from build123d import *

# Parameters (mm, degrees)
SKETCH1_R           = 21.5
SKETCH1_R_2         = 5
BOSS_EXTRUDE1_DEPTH = 5
EXTRUDE_THIN1_START = -100
SKETCH2_R           = 26.5
SKETCH2_R_2         = 21.5
EXTRUDE_THIN1_DEPTH = 100
CUT_EXTRUDE1_DEPTH  = 50
BOSS_EXTRUDE2_DEPTH = 5
SKETCH5_R           = 6
CUT_EXTRUDE2_DEPTH  = 5


with BuildPart() as part:
    # Sketch1 → Boss-Extrude1 (new body)
    with BuildSketch(Plane.XY):
        Circle(SKETCH1_R)
        Circle(SKETCH1_R_2, mode=Mode.SUBTRACT)
    extrude(amount=BOSS_EXTRUDE1_DEPTH)

    # Sketch2 → Extrude-Thin1 (add)
    with BuildSketch(Plane.XY.offset(5).offset(EXTRUDE_THIN1_START)):
        Circle(SKETCH2_R)
        Circle(SKETCH2_R_2, mode=Mode.SUBTRACT)
    extrude(amount=EXTRUDE_THIN1_DEPTH)

    # Sketch3 → Cut-Extrude1 (cut)
    with BuildSketch(Plane(origin=(0, 0, -95), x_dir=(-1, 0, 0), z_dir=(0, 0, -1))):
        with BuildLine():
            Line((11.936744149, -23.659335137), (11.494827009, -18.169175876))
            ThreePointArc((11.494827009, -18.169175876), (21.430686769, 1.725011487), (8.440695566, 19.773837725))
            Line((8.440695566, 19.773837725), (7.998778427, 25.263996985))
            ThreePointArc((7.998778427, 25.263996985), (26.414567412, 2.126176949), (11.936744149, -23.659335137))
        make_face()
        with BuildLine():
            Line((-11.494827009, 18.169175876), (-11.936744149, 23.659335137))
            ThreePointArc((-11.936744149, 23.659335137), (-26.414567412, -2.126176949), (-7.998778427, -25.263996985))
            Line((-7.998778427, -25.263996985), (-8.440695566, -19.773837725))
            ThreePointArc((-8.440695566, -19.773837725), (-21.430686769, -1.725011487), (-11.494827009, 18.169175876))
        make_face()
    extrude(amount=-CUT_EXTRUDE1_DEPTH, mode=Mode.SUBTRACT)

    # Sketch4 → Boss-Extrude2 (add)
    with BuildSketch(Plane(origin=(0, 0, -95), x_dir=(-1, 0, 0), z_dir=(0, 0, -1))):
        with BuildLine():
            Line((-11.494827009, 18.169175876), (-8.440695566, -19.773837725))
            ThreePointArc((-8.440695566, -19.773837725), (1.725011487, -21.430686769), (11.494827009, -18.169175876))
            Line((11.494827009, -18.169175876), (8.440695566, 19.773837725))
            ThreePointArc((8.440695566, 19.773837725), (-1.725011487, 21.430686769), (-11.494827009, 18.169175876))
        make_face()
    extrude(amount=-BOSS_EXTRUDE2_DEPTH)

    # Sketch5 → Cut-Extrude2 (cut)
    with BuildSketch(Plane(origin=(0, 0, -95), x_dir=(-1, 0, 0), z_dir=(0, 0, -1))):
        Circle(SKETCH5_R)
    extrude(amount=-CUT_EXTRUDE2_DEPTH, mode=Mode.SUBTRACT)


solid = part.part
Input: part model. Units: mm. Frame: model coordinates. A direction names the side the tool comes from. Coordinates: 2 decimals unless noted, no trailing zeros. Order: outer loops, then holes, each group sorted by start corner. A loop starts at its lowest first (then second) coordinate and runs counter-clockwise, first axis right, second up.
1. Draft query along Z for faces 1 (the cylindrical face through (-26.474, 1.165, -23.478)), 2 (the cylindrical face through (-21.48, 0.95, -25.63)), 3 (the flat face through (22, -1, -45)). Return one class per face: +Z half, -Z half, draft (parallel to the pull), parting line (faces both ways), or undercut.
Checked values:
face 1: draft
face 2: undercut
face 3: -Z half
2. Contact query for flat-ended pins moving along their axis: P1, Ø1, axis at x = 12.5, y = 13, coming from the -Z side; P2, Ø11, axis at x = 0, y = 0, coming from the +Z side; P3, Ø1, axis at x = -5.5, z = -27.5, coming from the -Y side; P4, Ø3, axis at y = -14.5, z = -18, coming from the +X side. Output: stop coordinate, or through.
Checked values:
P1: stops at z = 0
P2: stops at z = 5
P3: stops at y = -26.02
P4: stops at x = 23.09
3. Ray query, line 1 along Z through (x, y) = (4, 10); line 2 along Y through (x, z) = (0, -93); line 3 along Y through (x, z) = (0, -71). Return the intervals inside material, ascending.
Checked values:
line 1: z = -95 to -90, 0 to 5
line 2: y = -26.5 to -6, 6 to 26.5
line 3: y = -26.5 to -21.5, 21.5 to 26.5
4. Cut plane A-A, the plane z = -69. Return loops of the section in (x, y), plus the area to 3 significant figures.
Checked values:
outline: (-11.94, -23.66) arc R26.5 ccw to (8, -25.26) - (8.44, -19.77) arc R21.5 cw to (-11.49, -18.17) - close; (-8.44, 19.77) arc R21.5 cw to (11.49, 18.17) - (11.94, 23.66) arc R26.5 ccw to (-8, 25.26) - close
area: 206 mm2
5. Cut plane C-C, the plane y = -8. Return loops of the section in (x, z).
Checked values:
outline: (-25.26, -45) - (-19.96, -45) - (-19.96, 0) - (19.96, 0) - (19.96, -45) - (25.26, -45) - (25.26, 5) - (-25.26, 5) - close; (-10.68, -95) - (9.39, -95) - (9.39, -90) - (-10.68, -90) - close
6. Cut plane D-D, the plane y = 0. Return loops of the section in (x, z).
Checked values:
outline: (-26.5, -45) - (-21.5, -45) - (-21.5, 0) - (-5, 0) - (-5, 5) - (-26.5, 5) - close; (-10.03, -95) - (-6, -95) - (-6, -90) - (-10.03, -90) - close; (5, 0) - (21.5, 0) - (21.5, -45) - (26.5, -45) - (26.5, 5) - (5, 5) - close; (6, -95) - (10.03, -95) - (10.03, -90) - (6, -90) - close
7. Cut plane B-B, the plane x = 0. Return loops of the section in (y, z).
Checked values:
outline: (-26.5, -95) - (-6, -95) - (-6, -90) - (-21.5, -90) - (-21.5, 0) - (-5, 0) - (-5, 5) - (-26.5, 5) - close; (5, 0) - (21.5, 0) - (21.5, -90) - (6, -90) - (6, -95) - (26.5, -95) - (26.5, 5) - (5, 5) - close
8. Access query for faces 4 (the cylindrical face through (6, 0, -93)), 5 (the flat face through (4, -4, 0)), 6 (the flat face through (6, 0, 5)). Directions: +Z, -Z, +X, -X, +Y, -Y. A direction counts if a zero-diameter tool reaches every point of the face in a straight line with its end or side. Return the directions, or none.
Checked values:
face 4: -Z
face 5: none
face 6: +Z, +X, -X, +Y, -Y
